The figure shows three views and two pictorial views of one solid part (mm, origin at its lowest corner). Answer the questions. Coordinates: 2 decimals unless noted, no trailing zeros. Order: outer loops, then holes, each group sorted by start corner. A loop starts at its lowest first (then second) coordinate and runs counter-clockwise, first axis right, second up. Notation, with made-up numbers: M -13.75,-39 L 17.25,-39 A11 cw 17.25,-35 Z; hole C 23.5,-27.5 d5. An arc over 180 degrees is marked long. Answer in a Markdown table with one row per item. Add a question column.
Item 1: Flat-ended cylindrical pins translate along their axes: pin 1 Ø0.9 at (y, z) = (2, 56.5) entering from +X; pin 2 Ø1.5 at (x, y) = (15, 1.5) entering from -Z; pin 3 Ø2 at (x, z) = (3.5, 30.5) entering from -Y; pin 4 Ø1.5 at (y, z) = (1.5, 49) entering from -X. Find the tip coordinate at first contact, or state that the pin passes through.
Item 2: The part is cut by section C-C (x = 9). Write down the section's boundary in (y, z).
Item 3: Consider line 1 (Z direction, x = 20.75, y = 2.85); line 2 (X direction, y = 2.2, z = 4); line 3 (X direction, y = 2.55, z = 56). Determine where each line is inside the solid, lowest interval first. Write a range as from..to.
Item 4: The part is cut by section A-A (y = 0.95). Write down the section's boundary in (x, z), then the cut area to 3 significant figures.
Item 5: The part is cut by section B-B (z = 56.5). Write down the section's boundary in (x, y), then the cut area to 3 significant figures.
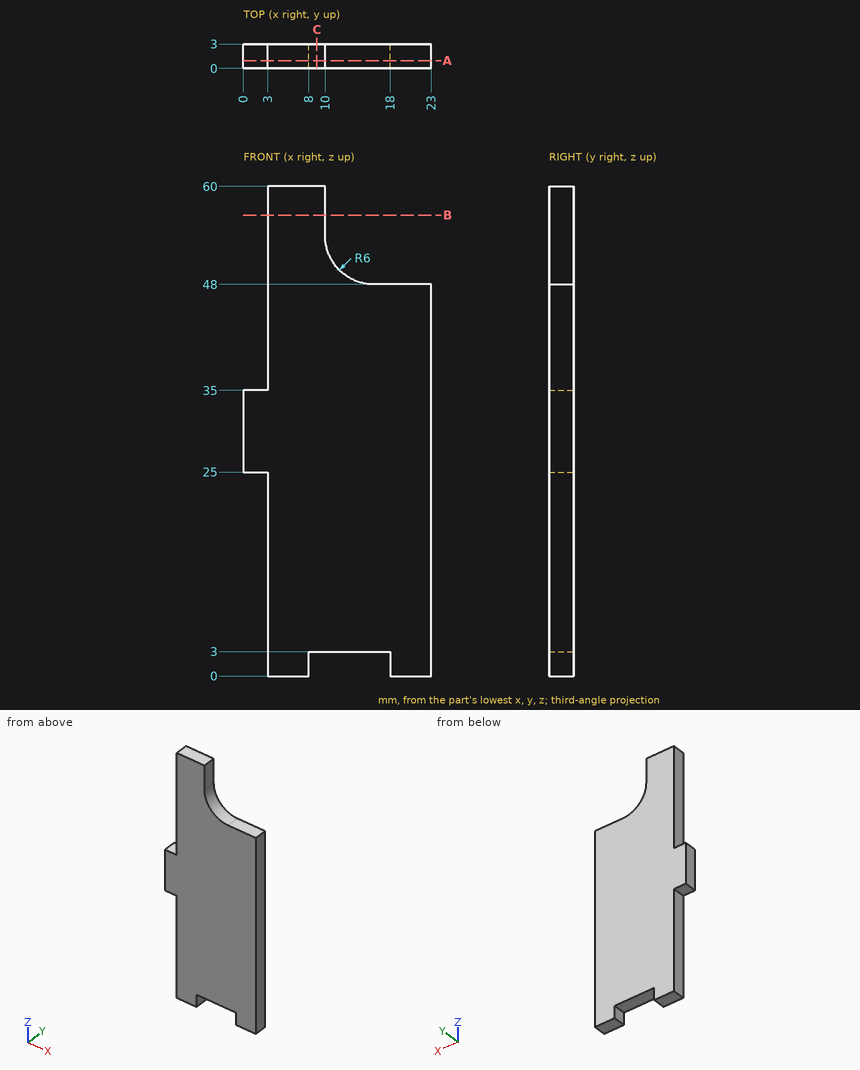
Reply:
| question | item | result |
|---|---|---|
| 1 | pin 1 | stops at x = 10 |
| 1 | pin 2 | stops at z = 3 |
| 1 | pin 3 | stops at y = 0 |
| 1 | pin 4 | stops at x = 3 |
| 2 | outline | M 0,3 L 3,3 L 3,60 L 0,60 Z |
| 3 | line 1 | z = 0..48 |
| 3 | line 2 | x = 3..23 |
| 3 | line 3 | x = 3..10 |
| 4 | outline | M 0,25 L 3,25 L 3,0 L 8,0 L 8,3 L 18,3 L 18,0 L 23,0 L 23,48 L 16,48 A6 cw 10,54 L 10,60 L 3,60 L 3,35 L 0,35 Z |
| 4 | area | 1,050 mm2 |
| 5 | outline | M 3,0 L 10,0 L 10,3 L 3,3 Z |
| 5 | area | 21.0 mm2 |
